Design review of the part built by this model. Coordinates are the model's own, in mm. Face numbers are marked on the shaded views. A direction names the side the tool comes from. Round coordinates to 2 decimals unless told otherwise and drop trailing zeros. Order: outer loops, then holes, each group sorted by start corner. A loop starts at its lowest first (then second) coordinate and runs counter-clockwise, first axis right, second up. Notation, with made-up numbers: M 74.25,1.25 L 124.25,1.25 A33 ccw 124.25,32.25 Z; hole C 48,-31 d9. An arc over 180 degrees is marked long. Write item = value, one per line. Start each with the question number.
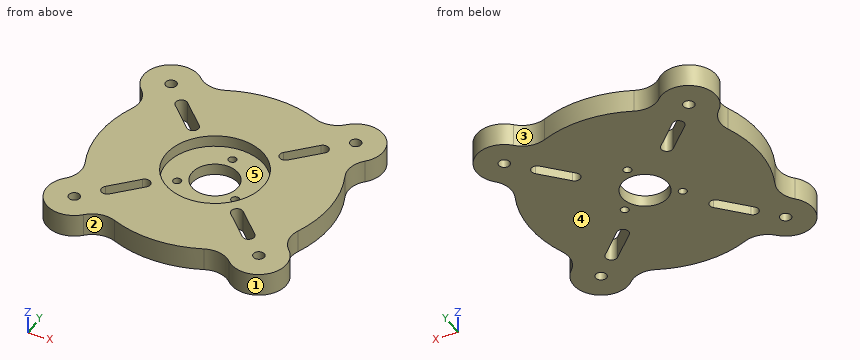
```python
from build123d import *

# Parameters (mm, degrees)
SKETCH1_R           = 2.4
SKETCH1_R_2         = 50
BOSS_EXTRUDE1_DEPTH = 10
SKETCH2_R           = 21.25
CUT_EXTRUDE1_DEPTH  = 5
SKETCH2_3_R         = 1.75
CUT_EXTRUDE2_DEPTH  = 75.1479844
SKETCH3_R           = 10
CUT_EXTRUDE3_DEPTH  = 74.640502379


with BuildPart() as part:
    # Sketch1 → Boss-Extrude1 (new body)
    # profile 1 of 5: a face of its own
    with BuildSketch(Plane.XY):
        with BuildLine():
            ThreePointArc((-31.466251763, -48.436814511), (-25.799706685, -45.41900176), (-19.413503243, -46.077281732))
            ThreePointArc((-19.413503243, -46.077281732), (-35.355339059, -35.355339059), (-46.077281732, -19.413503243))
            ThreePointArc((-46.077281732, -19.413503243), (-45.41900176, -25.799706685), (-48.436814511, -31.466251763))
            ThreePointArc((-48.436814511, -31.466251763), (-48.436814511, -48.436814511), (-31.466251763, -48.436814511))
        make_face()
        with Locations((-39.951533137, -39.951533137)):
            Circle(SKETCH1_R, mode=Mode.SUBTRACT)
    # profile 2 of 5: a face of its own
    with BuildSketch(Plane.XY):
        Circle(SKETCH1_R_2)
        with BuildLine():
            ThreePointArc((-28.838834765, 32.374368671), (-32.374368671, 32.374368671), (-32.374368671, 28.838834765))
            Line((-32.374368671, 28.838834765), (-21.767766953, 18.232233047))
            ThreePointArc((-21.767766953, 18.232233047), (-18.232233047, 18.232233047), (-18.232233047, 21.767766953))
            Line((-18.232233047, 21.767766953), (-28.838834765, 32.374368671))
        make_face(mode=Mode.SUBTRACT)
        with BuildLine():
            ThreePointArc((-32.374368671, -28.838834765), (-32.374368671, -32.374368671), (-28.838834765, -32.374368671))
            Line((-28.838834765, -32.374368671), (-18.232233047, -21.767766953))
            ThreePointArc((-18.232233047, -21.767766953), (-18.232233047, -18.232233047), (-21.767766953, -18.232233047))
            Line((-21.767766953, -18.232233047), (-32.374368671, -28.838834765))
        make_face(mode=Mode.SUBTRACT)
        with BuildLine():
            ThreePointArc((28.838834765, -32.374368671), (32.374368671, -32.374368671), (32.374368671, -28.838834765))
            Line((32.374368671, -28.838834765), (21.767766953, -18.232233047))
            ThreePointArc((21.767766953, -18.232233047), (18.232233047, -18.232233047), (18.232233047, -21.767766953))
            Line((18.232233047, -21.767766953), (28.838834765, -32.374368671))
        make_face(mode=Mode.SUBTRACT)
        with BuildLine():
            ThreePointArc((32.374368671, 28.838834765), (32.374368671, 32.374368671), (28.838834765, 32.374368671))
            Line((28.838834765, 32.374368671), (18.232233047, 21.767766953))
            ThreePointArc((18.232233047, 21.767766953), (18.232233047, 18.232233047), (21.767766953, 18.232233047))
            Line((21.767766953, 18.232233047), (32.374368671, 28.838834765))
        make_face(mode=Mode.SUBTRACT)
    # profile 3 of 5: a face of its own
    with BuildSketch(Plane.XY):
        with BuildLine():
            ThreePointArc((-46.077281732, 19.413503243), (-35.355339059, 35.355339059), (-19.413503243, 46.077281732))
            ThreePointArc((-19.413503243, 46.077281732), (-25.799706685, 45.41900176), (-31.466251763, 48.436814511))
            ThreePointArc((-31.466251763, 48.436814511), (-48.436814511, 48.436814511), (-48.436814511, 31.466251763))
            ThreePointArc((-48.436814511, 31.466251763), (-45.41900176, 25.799706685), (-46.077281732, 19.413503243))
        make_face()
        with Locations((-39.951533137, 39.951533137)):
            Circle(SKETCH1_R, mode=Mode.SUBTRACT)
    # profile 4 of 5: a face of its own
    with BuildSketch(Plane.XY):
        with BuildLine():
            ThreePointArc((19.413503243, 46.077281732), (35.355339059, 35.355339059), (46.077281732, 19.413503243))
            ThreePointArc((46.077281732, 19.413503243), (45.41900176, 25.799706685), (48.436814511, 31.466251763))
            ThreePointArc((48.436814511, 31.466251763), (48.436814511, 48.436814511), (31.466251763, 48.436814511))
            ThreePointArc((31.466251763, 48.436814511), (25.799706685, 45.41900176), (19.413503243, 46.077281732))
        make_face()
        with Locations((39.951533137, 39.951533137)):
            Circle(SKETCH1_R, mode=Mode.SUBTRACT)
    # profile 5 of 5: a face of its own
    with BuildSketch(Plane.XY):
        with BuildLine():
            ThreePointArc((48.436814511, -31.466251763), (45.41900176, -25.799706685), (46.077281732, -19.413503243))
            ThreePointArc((46.077281732, -19.413503243), (35.355339059, -35.355339059), (19.413503243, -46.077281732))
            ThreePointArc((19.413503243, -46.077281732), (25.799706685, -45.41900176), (31.466251763, -48.436814511))
            ThreePointArc((31.466251763, -48.436814511), (48.436814511, -48.436814511), (48.436814511, -31.466251763))
        make_face()
        with Locations((39.951533137, -39.951533137)):
            Circle(SKETCH1_R, mode=Mode.SUBTRACT)
    extrude(amount=BOSS_EXTRUDE1_DEPTH)

    # Sketch2 → Cut-Extrude1 (cut)
    with BuildSketch(Plane.XY.offset(10)):
        Circle(SKETCH2_R)
    extrude(amount=-CUT_EXTRUDE1_DEPTH, mode=Mode.SUBTRACT)

    # Sketch2_3 → Cut-Extrude2 (cut, through all)
    with BuildSketch(Plane.XY.offset(10)):
        with Locations((0, 14.5)):
            Circle(SKETCH2_3_R)
        with Locations((12.557368355, -7.25)):
            Circle(SKETCH2_3_R)
        with Locations((-12.557368355, -7.25)):
            Circle(SKETCH2_3_R)
    extrude(amount=-CUT_EXTRUDE2_DEPTH, mode=Mode.SUBTRACT)

    # Sketch3 → Cut-Extrude3 (cut, through all)
    with BuildSketch(Plane.XY.offset(5)):
        Circle(SKETCH3_R)
    extrude(amount=-CUT_EXTRUDE3_DEPTH, mode=Mode.SUBTRACT)


solid = part.part
```
(1) Insertion check: pin 1 (6 mm diameter, centred on x = 27, z = 1.5, fed in from +Y); pin 2 (3 mm diameter, centred on x = 0, y = 14.5, fed in from +Z) (3 decimals); pin 3 (2 mm diameter, centred on x = 0.5, z = 5.5, fed in from -Y); pin 4 (4 mm diameter, centred on x = -24, z = 5.5, fed in from -Y). Each pin has a flat end and moves straight along its axis. Give the tip position at first contact, or say it passes through.
(2) Consider section B-B, the plane y = 0. Write out the cut boundary in (x, z), then the cut area to 4 significant figures.
(3) Draft analysis for pull direction Y (two halves, no side actions). For the marked faces 1, 2 and 3, state which applies: pulls with the +Y half, pulls with the -Y half, needs draft (parallel to the pull), parting line crosses it, or undercut.
(4) For line 1 along Y through (x, z) = (0, 3.9); line 2 along X through (y, z) = (-40, 9); line 3 along Y through (x, z) = (-23, 2.5), list the stretches that pass through material, from the lowest coordinate up. Write a range as [from, to].
(5) Consider section C-C, the plane y = -25.5. Write out the cut boundary in (x, z), then the cut area to 3 significant figures.
(6) Consider section A-A, the plane x = 0. Write out the cut boundary in (y, z).
(7) For the marked faces 4 and 5, list the 3-axis set-ups (+Z, -Z, +X, -X, +Y, -Y) from which the entire face can be reached by the end or side of a thin tool; tool diameter is ignored.
(8) Consider section D-D, the plane x = -25. Write out the cut boundary in (y, z), then the cut area to 3 significant figures.
Completed:
q1.pin_1 = 47.21
q1.pin_2 = through
q1.pin_3 = -50
q1.pin_4 = -45.46
q2.outline = M -50,0 L -10,0 L -10,5 L -21.25,5 L -21.25,10 L -50,10 Z; M 10,0 L 50,0 L 50,10 L 21.25,10 L 21.25,5 L 10,5 Z
q2.area = 687.5 mm2
q3.face_1 = undercut
q3.face_2 = pulls with the -Y half
q3.face_3 = pulls with the +Y half
q4.line_1 = [-50, -10], [10, 12.75], [16.25, 50]
q4.line_2 = [-51.95, -42.35], [-37.55, 37.55], [42.35, 51.95]
q4.line_3 = [-45.24, -26.54], [-19.46, 19.46], [26.54, 45.24]
q5.outline = M -45.36,0 L -29.04,0 L -29.04,10 L -45.36,10 Z; M -21.96,0 L 21.96,0 L 21.96,10 L -21.96,10 Z; M 29.04,0 L 45.36,0 L 45.36,10 L 29.04,10 Z
q5.area = 766 mm2
q6.outline = M -50,0 L -10,0 L -10,5 L -21.25,5 L -21.25,10 L -50,10 Z; M 10,0 L 12.75,0 L 12.75,5 L 10,5 Z; M 16.25,0 L 50,0 L 50,10 L 21.25,10 L 21.25,5 L 16.25,5 Z
q7.face_4 = -Z, +X, -X, +Y, -Y
q7.face_5 = +Z
q8.outline = M -45.29,0 L -28.54,0 L -28.54,10 L -45.29,10 Z; M -21.46,0 L 21.46,0 L 21.46,10 L -21.46,10 Z; M 28.54,0 L 45.29,0 L 45.29,10 L 28.54,10 Z
q8.area = 764 mm2
